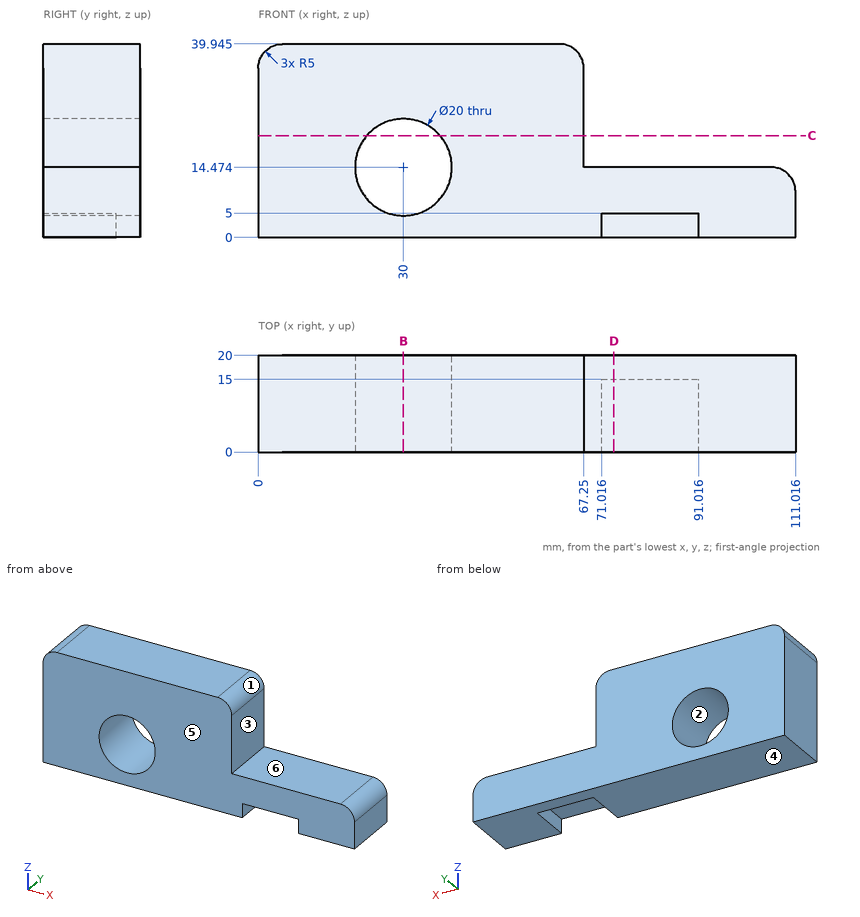
For this review, use the dimensioned drawing (mm, ordinates from the lowest corner) and the shaded views. A direction names the side the tool comes from. Give positions to 0.01 mm unless a question says otherwise; leave off trailing zeros. Order: outer loops, then holes, each group sorted by start corner. A loop starts at its lowest first (then second) coordinate and runs counter-clockwise, first axis right, second up. Notation, with made-up numbers: (-27.75, 34.25) - (-23.75, 34.25) arc R9 ccw to (-23.75, 46.25) - close; hole circle Ø4 at (-26, 6.5). An arc over 180 degrees is marked (long way). Use CSV: the item, a comma, the result in double quotes. Start each with the question number.
Q1. For line 1 (Z direction, x = 30, y = 14.75) (1 decimal); line 2 (Z direction, x = 82, y = 19.25); line 3 (X direction, y = 3, z = 7) (1 decimal), list the stretches that pass through material, from the lowest coordinate up.
Q2. Take a section at C-C (z = 21). State the section outline as (x, y) points, and give its area (3 significant figures).
Q3. Take a section at D-D (x = 73.5). State the section outline as (y, z) points.
Q4. For P1, Ø10, axis at x = 91, y = 11.5, coming from the +Z side; P2, Ø1.5, axis at x = 84, z = 2.5, coming from the -Y side; P3, Ø7.5, axis at x = 83, y = 5, coming from the -Z side, all flat-tipped, find the tip position at first contact; note any pin that passes through.
Q5. Take a section at B-B (x = 30). State the section outline as (y, z) points (1 decimal), and give its area (3 significant figures).
Q6. Draft analysis for pull direction Z (two halves, no side actions). For the marked faces 1, 2, 3 and 4, state which applies: pulls with the +Z half, pulls with the -Z half, needs draft (parallel to the pull), parting line crosses it, or undercut.
Q7. Machinability: for the marked faces 5 and 6, which of the approach directions +Z, -Z, +X, -X, +Y, -Y give a long, thin tool a straight path to every point of the face, cutting with its end or side? Answer none if there is none.
Calculated:
1,line 1,"z = 0 to 4.5, 24.5 to 39.9"
1,line 2,"z = 0 to 14.47"
1,line 3,"x = 0 to 23.4, 36.6 to 111"
2,outline,"(0, 0) - (22.42, 0) - (22.42, 20) - (0, 20) - close; (37.58, 0) - (67.25, 0) - (67.25, 20) - (37.58, 20) - close"
2,area,"1,040 mm²"
3,outline,"(0, 5) - (15, 5) - (15, 0) - (20, 0) - (20, 14.47) - (0, 14.47) - close"
4,P1,"stops at z = 14.47"
4,P2,"stops at y = 15"
4,P3,"stops at z = 5"
5,outline,"(0, 0) - (20, 0) - (20, 4.5) - (0, 4.5) - close; (0, 24.5) - (20, 24.5) - (20, 39.9) - (0, 39.9) - close"
5,area,"399 mm²"
6,face 1,"pulls with the +Z half"
6,face 2,"undercut"
6,face 3,"needs draft"
6,face 4,"pulls with the -Z half"
7,face 5,"+Z, -Z, +X, -X, -Y"
7,face 6,"+Z, +X, +Y, -Y"
